Check sheet for the modelled part. Datum: model origin and axes. Units: mm. A direction names the side the tool comes from. Give positions to 0.01 mm unless a question says otherwise; leave off trailing zeros. Order: outer loops, then holes, each group sorted by start corner. A loop starts at its lowest first (then second) coordinate and runs counter-clockwise, first axis right, second up. Notation, with made-up numbers: (11, 52.25) -> (36, 52.25) arc R19 ccw to (36, 75.25) -> close; hole circle Ø6 at (76, 75). An arc over 180 degrees is marked (long way). Answer in a Markdown table with one row per item. Add a question column.
(1) Cross-section at A-A (z = 5.75). Record the cut outline in (x, y), then the cut area to 3 significant figures.
(2) Cross-section at B-B (y = 4.5). Record the cut outline in (x, z).
(3) Release check for a two-part mould opening along Z. For faces 3 (the face through (4.783, -0.14, 3.428)), 4 (the face through (0, -11.5, 3)), 5 (the face through (0, 0, 0)) record: released by +Z, released by -Z, zero draft, split by the parting line, or undercut.
(4) Cross-section at C-C (x = -5.75). Record the cut outline in (y, z).
(5) Go/stop test with flat-tipped pins: pin 1 (4 mm diameter, centred on y = 5.5, z = 7.5, fed in from -X); pin 2 (1.5 mm diameter, centred on y = -4.5, z = 7, fed in from -X); pin 3 (8 mm diameter, centred on x = -6, y = 7, fed in from +Z); pin 4 (5 mm diameter, centred on y = -7.5, z = 7.5, fed in from -X). Record where each tip stops, or that it passes through.
(6) Cross-section at D-D (z = 2.75). Record the cut outline in (x, y).
(7) Set-up check for faces 1 (the face through (-6.295, -0.14, 3.047)), 2 (the face through (-6.03, -0.16, 7.15)): record each of +Z, -Z, +X, -X, +Y, -Y from which the full face is reachable in a straight line by a thin tool's end or side.
(8) Thickness scan on L1, parallel to Y at x = 7.25, z = 5; L2, parallel to X at y = 9.75, z = 1.75; L3, parallel to X at y = 9.5, z = 3.5. Record the ranges inside material, lowest first. Write a range as [from, to].
```python
from build123d import *

# Parameters (mm, degrees)
F2_DEPTH = 11.5
F4_W     = 1.5
F4_H     = 20
F5_DEPTH = 25
F6_R     = 0.25


with BuildPart() as f2:
    # F1 (on Front) → F2 (new body, symmetric)
    with BuildSketch(Plane.XZ):
        with BuildLine():
            Line((-10.6042210982, 4.5106432563), (-8, 0))
            Line((-8, 0), (0, 0))
            Line((0, 0), (0, 5))
            ThreePointArc((0, 5), (-2.4494897428, 6.2679491924), (-2.8284271247, 9))
            Line((-2.8284271247, 9), (-10.6042210982, 4.5106432563))
        make_face()
    extrude(amount=F2_DEPTH, both=True)

    # F4 (on offset) → F5 (cut)
    with BuildSketch(Plane(origin=(-4.6042210982, 0, 7.9747448714), x_dir=(0.8660254038, 0, 0.5), z_dir=(-0.5, 0, 0.8660254038))):
        with Locations((-3.1782032303, 0)):
            Rectangle(F4_W, F4_H)
    extrude(amount=-F5_DEPTH, mode=Mode.SUBTRACT)

    # F6
    f6_edges = [f2.edges().sort_by_distance(p)[0] for p in [
        (-10.604221, 0, 4.510643),
        (-2.828427, 0, 9),
    ]]
    fillet(f6_edges, radius=F6_R)

    # F7: F2 across plane


with BuildPart() as f2_1:
    add(f2.part)
    add(f2.part.mirror(Plane.YZ))


solid = f2_1.part
```
Answer below:
| question | item | result |
|---|---|---|
| 1 | outline | (-8.46, -11.5) -> (-1.98, -11.5) -> (-1.98, 11.5) -> (-8.46, 11.5) -> close; (1.98, -11.5) -> (8.46, -11.5) -> (8.46, 11.5) -> (1.98, 11.5) -> close; hole (-7.86, -10) -> (-6.12, -10) -> (-6.12, 10) -> (-7.86, 10) -> close; hole (6.12, -10) -> (7.86, -10) -> (7.86, 10) -> (6.12, 10) -> close |
| 1 | area | 228 mm² |
| 2 | outline | (-10.48, 4.29) -> (-8, 0) -> (-4.54, 0) -> (-8.01, 6.01) -> (-10.39, 4.64) arc R0.25 ccw to start; (-6.71, 6.76) -> (-2.8, 0) -> (2.8, 0) -> (6.71, 6.76) -> (3.34, 8.71) arc R0.25 ccw to (2.97, 8.45) arc R3 cw (long way) to (-2.97, 8.45) arc R0.25 ccw to (-3.34, 8.71) -> close; (4.54, 0) -> (8, 0) -> (10.48, 4.29) arc R0.25 ccw to (10.39, 4.64) -> (8.01, 6.01) -> close |
| 3 | face 3 | undercut |
| 3 | face 4 | zero draft |
| 3 | face 5 | released by -Z |
| 4 | outline | (-11.5, 0) -> (11.5, 0) -> (11.5, 7.31) -> (-11.5, 7.31) -> close; hole (-10, 2.1) -> (10, 2.1) -> (10, 5.1) -> (-10, 5.1) -> close |
| 5 | pin 1 | stops at x = -8.89 |
| 5 | pin 2 | stops at x = -6.71 |
| 5 | pin 3 | stops at z = 8.74 |
| 5 | pin 4 | stops at x = -9.76 |
| 6 | outline | (-9.59, -11.5) -> (9.59, -11.5) -> (9.59, 11.5) -> (-9.59, 11.5) -> close; hole (-6.12, -10) -> (-4.39, -10) -> (-4.39, 10) -> (-6.12, 10) -> close; hole (4.39, -10) -> (6.12, -10) -> (6.12, 10) -> (4.39, 10) -> close |
| 7 | face 1 | none |
| 7 | face 2 | +Z, -X, +Y, -Y |
| 8 | L1 | y = [-11.5, -10], [10, 11.5] |
| 8 | L2 | x = [-9.01, -5.55], [-3.81, 3.81], [5.55, 9.01] |
| 8 | L3 | x = [-10.02, -6.56], [-4.82, 4.82], [6.56, 10.02] |
